Can you work these out from the model? Positions are in its coordinate system, mm. Round coordinates to 2 decimals unless told otherwise and drop trailing zeros. Order: outer loops, then holes, each group sorted by start corner. A loop starts at its lowest first (then second) coordinate and runs counter-clockwise, first axis right, second up.
Q1. If I drill on line 1 (X direction, y = 169, z = 10.5); line 2 (X direction, y = 582.5, z = 1.25); line 3 (Y direction, x = 434, z = 4.25), over which ranges is the centre line in solid material (lowest first)?
Q2. If we section it at C-C (z = 4.75): Please give me the cut outline in (x, y), plus the area to 3 significant figures.
Q3. If we section it at A-A (x = 250): Please give me the cut outline in (y, z), plus the area to 3 significant figures.
Q4. If we section it at B-B (y = 257.5): Please give me the cut outline in (x, z).
Q5. Will these pins go through, and if not, where does the flat tip stop? P1, Ø1, axis at x = 148, z = 10, coming from the +Y side; P2, Ø5, axis at y = 624.5, z = 8, coming from the -X side; P3, Ø1.6, axis at x = 0.5, z = 9, coming from the +Y side.
Solid Edge part; units mm, degrees
sketch "Sketch1" plane through (0, 0, 0) normal (0, 0, 1) x (1, 0, 0)
  line L0 (0, 0) -> (500, 0)
  line L1 (500, 0) -> (500, 550)
  arc A0 (0, 550) -> (500, 550) centre (250, 550) cw
  line L2 (0, 550) -> (0, 0)
extrude "Protrusion1" add sketch "Sketch1" along normal blind 12
sketch "Sketch2" plane through (250, 400, 0) normal (0, 0, -1) x (-1, 0, 0)
  line L0 (250, 150) -> (248, 150)
  arc A0 (-248, 150) -> (248, 150) centre (0, 150) cw
  line L1 (-250, 150) -> (-248, 150)
  arc A1 (250, 150) -> (-250, 150) centre (0, 150) ccw
extrude "Ausschnitt_6" cut sketch "Sketch2" against normal blind 184.2167
sketch "Sketch3" plane through (250, 399, 0) normal (0, 0, -1) x (-1, 0, 0)
  line L0 (-200, -349) -> (200, -349)
  line L1 (200, -349) -> (200, 151)
  arc A0 (-200, 151) -> (200, 151) centre (0, 151) cw
  line L2 (-200, 151) -> (-200, -349)
  dimension "D1" = 200
  dimension "D2" = 200
extrude "Ausschnitt_7" cut sketch "Sketch3" against normal blind 568.3558
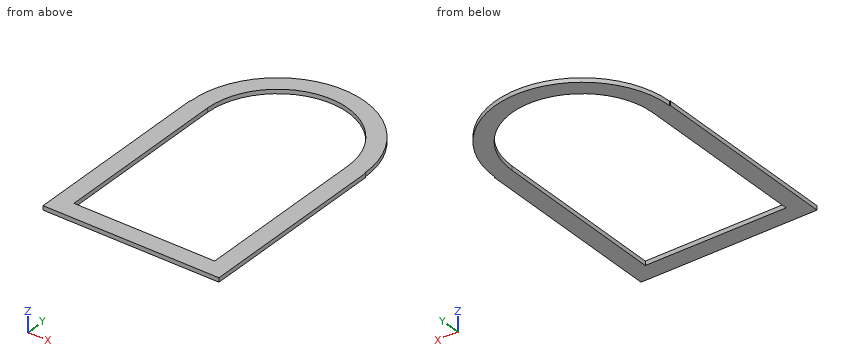
Solution:
1. line 1: x = 0 to 50, 450 to 500
1. line 2: x = 4.14 to 52.66, 447.34 to 495.86
1. line 3: y = 0 to 50, 628.38 to 716.28
2. outline: (0, 0) - (500, 0) - (500, 550) - (498, 550) arc R248 ccw to (2, 550) - (0, 550) - close; hole (50, 50) - (450, 50) - (450, 550) arc R200 ccw to (50, 550) - close
2. area: 109,000 mm2
3. outline: (0, 0) - (50, 0) - (50, 12) - (0, 12) - close; (750, 0) - (798, 0) - (798, 12) - (750, 12) - close
3. area: 1,180 mm2
4. outline: (0, 0) - (50, 0) - (50, 12) - (0, 12) - close; (450, 0) - (500, 0) - (500, 12) - (450, 12) - close
5. P1: stops at y = 776.28
5. P2: stops at x = 12.68
5. P3: stops at y = 550
